```python
from build123d import *

# Parameters (mm, degrees)
BOSS_EXTRUDE1_DEPTH = 10
FILLET1_R           = 0.025
FILLET2_R           = 0.05


with BuildPart() as part:
    # Sketch1 → Boss-Extrude1 (new body)
    with BuildSketch(Plane.XY):
        with BuildLine():
            ThreePointArc((2, -2.5), (0, -4.5), (-2, -2.5))
            Line((-2, -2.5), (-2, 2.5))
            ThreePointArc((-2, 2.5), (0, 4.5), (2, 2.5))
            add(Edge.make_bspline(
                [(2, 2.5), (2.759271996, 1.299931224), (3, 0)],
                knots=[0, 0, 0, 0.518543991, 0.518543991, 0.518543991], degree=2))
            Line((3, 0), (3, 2.5))
            ThreePointArc((3, 2.5), (0, 5.5), (-3, 2.5))
            Line((-3, 2.5), (-3, -2.5))
            ThreePointArc((-3, -2.5), (0, -5.5), (3, -2.5))
            add(Edge.make_bspline(
                [(3, -2.5), (2.709402649, 0.136566945), (1.5, 2.5)],
                knots=[0, 0, 0, 1, 1, 1], degree=2))
            add(Edge.make_bspline(
                [(2, -2.5), (2.245145169, 0.049029034), (1.5, 2.5)],
                knots=[0, 0, 0, 1, 1, 1], degree=2))
        make_face()
    extrude(amount=BOSS_EXTRUDE1_DEPTH)

    # Fillet1
    fillet1_edges = [part.edges().sort_by_distance(p)[0] for p in [
        (1.5, 2.5, 5),
    ]]
    fillet(fillet1_edges, radius=FILLET1_R)

    # Fillet2
    fillet2_edges = [part.edges().sort_by_distance(p)[0] for p in [
        (3, 0, 5),
    ]]
    fillet(fillet2_edges, radius=FILLET2_R)


solid = part.part
```
Can you work these out from the model? Positions are in its coordinate system, mm. A direction names the side the tool comes from. Round coordinates to 2 decimals unless told otherwise and drop trailing zeros. Loops run counter-clockwise (first coordinate to the right, second up) from the corner with the lowest first, then second, coordinate; pieces in that order, holes last. Notation, with made-up numbers: (56, 80) -> (115, 80) arc R8 cw to (115, 94) -> close; hole circle Ø9 at (-25.5, 33). An arc over 180 degrees is marked (long way). Answer in a Markdown table with one row per item.
Item 1: Will these pins go through, and if not, where does the flat tip stop? P1, Ø2, axis at y = -4, z = 3.5, coming from the -X side; P2, Ø1.5, axis at x = -2, z = 7.5, coming from the -Y side.
Answer block:
| item | result |
|---|---|
| P1 | x = -2.96 |
| P2 | y = -5.23 |
Item 2: We'd pull the mould along X, two halves only. Please class faces 3 (the cylindrical face through (0, 4.5, 4.9)), 4 (the cylindrical face through (-0.1, -5.5, 4.9)), 5 (the flat face through (3, 1, 5)), 6 (the flat face through (-2, 0, 5)): released by +X, released by -X, zero draft, split by the parting line, or undercut.
Answer block:
| item | result |
|---|---|
| face 3 | undercut |
| face 4 | split by the parting line |
| face 5 | released by +X |
| face 6 | undercut |
Item 3: Suppose I cut it at A-A, the plane x = 0. List the corners of the cut face in (y, z) for me.
Answer block:
| item | result |
|---|---|
| outline | (-5.5, 0) -> (-4.5, 0) -> (-4.5, 10) -> (-5.5, 10) -> close; (4.5, 0) -> (5.5, 0) -> (5.5, 10) -> (4.5, 10) -> close |
Item 4: Suppose I cut it at C-C, the plane y = 2. Give the number of separate pieces and of enclosed holes in the cut face, plus the area to 3 significant figures.
Answer block:
| item | result |
|---|---|
| separate pieces | 3 |
| enclosed holes | 0 |
| area | 18.1 mm² |
Item 5: If I drill on probe 1 along Y at (x, z) = (0, 6); probe 2 along X at (y, z) = (-2.5, 1); probe 3 along Y at (x, z) = (-0.5, 3.25), over which ranges is the centre line in solid material (lowest first)?
Answer block:
| item | result |
|---|---|
| probe 1 | -5.5 to -4.5, 4.5 to 5.5 |
| probe 2 | -3 to -2, 2 to 3 |
| probe 3 | -5.46 to -4.44, 4.44 to 5.46 |
Item 6: Suppose I cut it at B-B, the plane y = 4. List the corners of the cut face in (x, z) for me, plus the area to 3 significant figures.
Answer block:
| item | result |
|---|---|
| outline | (-2.6, 0) -> (-1.32, 0) -> (-1.32, 10) -> (-2.6, 10) -> close; (1.32, 0) -> (2.6, 0) -> (2.6, 10) -> (1.32, 10) -> close |
| area | 25.5 mm² |
Item 7: On a 3-axis mill with a long thin cutter (end or side, diameter ignored), from which of +Z, -Z, +X, -X, +Y, -Y can I reach the whole of each face in a straight line? I mean faces 1 (the cylindrical face through (0, -4.5, 4.9)), 2 (the flat face through (-2.7, 0.1, 0)). Say none if no direction works.
Answer block:
| item | result |
|---|---|
| face 1 | +Z, -Z |
| face 2 | -Z, +X, -X, +Y, -Y |
